Read the model definition and answer for the solid it produces. Units are mm, in the model's axes. Face numbers are marked on the shaded views. A direction names the side the tool comes from. Coordinates: 2 decimals unless noted, no trailing zeros. Write each loop counter-clockwise with the first axis right and the second up, starting at its lowest first coordinate (ties: lowest second). Pieces come first, ordered by that corner, then holes. Notation, with made-up numbers: (14, 89.5) - (55, 89.5) arc R25 cw to (55, 117.5) - close; hole circle Ø8 at (4.25, 76.25). An arc over 180 degrees is marked (long way). Return JSON: item names as keys, results as strings.
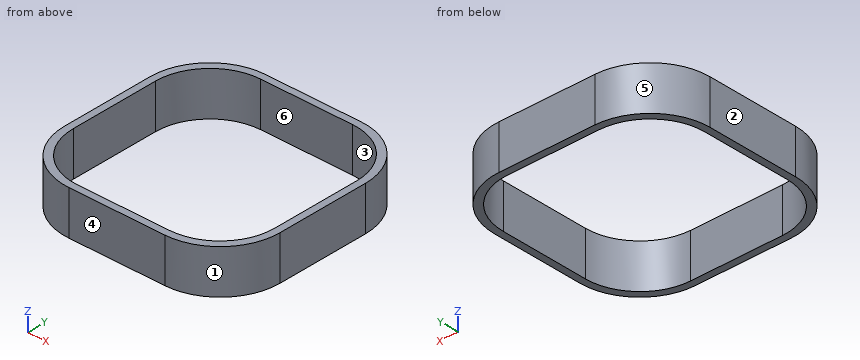
```python
from build123d import *

# Parameters (mm, degrees)
BOX001_W     = 114.5
BOX001_H     = 112.5
BOX001_DEPTH = 32
BOX_W        = 122.5
BOX_H        = 120.5
BOX_DEPTH    = 25
FILLET_R     = 31
FILLET001_R  = 31
FILLET002_R  = 31
FILLET003_R  = 31
FILLET004_R  = 34
FILLET005_R  = 34
FILLET009_R  = 34
FILLET008_R  = 34


with BuildPart() as cubo001:
    # Box001 → Box001 (new body)
    with BuildSketch(Plane(origin=(4, 4, 0), x_dir=(1, 0, 0), z_dir=(0, 0, 1))):
        with Locations((57.25, 56.25)):
            Rectangle(BOX001_W, BOX001_H)
    extrude(amount=BOX001_DEPTH)


with BuildPart() as fillet008:
    # Box → Box (new body)
    with BuildSketch(Plane.XY):
        with Locations((61.25, 60.25)):
            Rectangle(BOX_W, BOX_H)
    extrude(amount=BOX_DEPTH)

    # Cut: cut Cubo001
    add(cubo001.part, mode=Mode.SUBTRACT)

    # Fillet
    fillet_edges = [fillet008.edges().sort_by_distance(p)[0] for p in [
        (4, 116.5, 12.5),
    ]]
    fillet(fillet_edges, radius=FILLET_R)

    # Fillet001
    fillet001_edges = [fillet008.edges().sort_by_distance(p)[0] for p in [
        (118.5, 116.5, 12.5),
    ]]
    fillet(fillet001_edges, radius=FILLET001_R)

    # Fillet002
    fillet002_edges = [fillet008.edges().sort_by_distance(p)[0] for p in [
        (4, 4, 12.5),
    ]]
    fillet(fillet002_edges, radius=FILLET002_R)

    # Fillet003
    fillet003_edges = [fillet008.edges().sort_by_distance(p)[0] for p in [
        (118.5, 4, 12.5),
    ]]
    fillet(fillet003_edges, radius=FILLET003_R)

    # Fillet004
    fillet004_edges = [fillet008.edges().sort_by_distance(p)[0] for p in [
        (0, 120.5, 12.5),
    ]]
    fillet(fillet004_edges, radius=FILLET004_R)

    # Fillet005
    fillet005_edges = [fillet008.edges().sort_by_distance(p)[0] for p in [
        (122.5, 120.5, 12.5),
    ]]
    fillet(fillet005_edges, radius=FILLET005_R)

    # Fillet009
    fillet009_edges = [fillet008.edges().sort_by_distance(p)[0] for p in [
        (122.5, 0, 12.5),
    ]]
    fillet(fillet009_edges, radius=FILLET009_R)

    # Fillet008
    fillet008_edges = [fillet008.edges().sort_by_distance(p)[0] for p in [
        (0, 0, 12.5),
    ]]
    fillet(fillet008_edges, radius=FILLET008_R)


solid = fillet008.part
```
(1) Determine the mould class of the marked faces 1, 2, 3 and 4 for opening direction X: +X half, -X half, draft (parallel to the pull), parting line (faces both ways), or undercut.
Answer:
{"face 1": "+X half", "face 2": "-X half", "face 3": "undercut", "face 4": "draft"}
(2) A cutting plane is placed at C-C (z = 9.5). Determine the outline of the cut face in (x, y).
Answer:
{"outline": "(0, 34) arc R34 ccw to (34, 0) - (88.5, 0) arc R34 ccw to (122.5, 34) - (122.5, 86.5) arc R34 ccw to (88.5, 120.5) - (34, 120.5) arc R34 ccw to (0, 86.5) - close; hole (4, 35) arc R31 ccw to (35, 4) - (87.5, 4) arc R31 ccw to (118.5, 35) - (118.5, 85.5) arc R31 ccw to (87.5, 116.5) - (35, 116.5) arc R31 ccw to (4, 85.5) - close"}
(3) Straight lines are drawn through the part: line 1 (Y direction, x = 53, z = 6.25); line 2 (X direction, y = 84, z = 8); line 3 (X direction, y = 112.5, z = 20). For each, find the intervals that lie inside material, in ascending order. Write a range as from..to.
Answer:
{"line 1": "0..4, 116.5..120.5", "line 2": "0..4, 118.5..122.5", "line 3": "12.09..19.77, 102.73..110.41"}
(4) Which of the six approach directions +Z, -Z, +X, -X, +Y, -Y give full straight-line access (tool end or side, diameter ignored) to the marked faces 5 and 6?
Answer:
{"face 5": "+Z, -Z, -X, +Y", "face 6": "+Z, -Z"}
(5) Flat-ended cylindrical pins translate along their axes: P1, Ø3, axis at y = 89.5, z = 19.5, coming from the +X side; P2, Ø1, axis at y = 31, z = 8, coming from the +X side; P3, Ø1.5, axis at y = 19.5, z = 20, coming from the -X side. Find the tip coordinate at first contact, or state that the pin passes through.
Answer:
{"P1": "x = 122.47", "P2": "x = 122.41", "P3": "x = 2.9"}
(6) A cutting plane is placed at A-A (y = 55.5). Determine the outline of the cut face in (x, z).
Answer:
{"outline": "(0, 0) - (4, 0) - (4, 25) - (0, 25) - close; (118.5, 0) - (122.5, 0) - (122.5, 25) - (118.5, 25) - close"}
(7) A cutting plane is placed at B-B (x = 77.5). Determine the outline of the cut face in (y, z), and give its area (3 significant figures).
Answer:
{"outline": "(0, 0) - (4, 0) - (4, 25) - (0, 25) - close; (116.5, 0) - (120.5, 0) - (120.5, 25) - (116.5, 25) - close", "area": "200 mm²"}
